```python
from build123d import *

# Parameters (mm, degrees)
ESQUISSE1_R             = 50
BOSS_EXTRU_1_DEPTH      = 10
ESQUISSE2_R             = 47.5
ENL_V_MAT_EXTRU_1_DEPTH = 5
ESQUISSE3_R             = 2
ENL_V_MAT_EXTRU_2_DEPTH = 5
BOSS_EXTRU_2_DEPTH      = 100
CONG_1_R                = 30
ESQUISSE5_R             = 12.5
BOSS_EXTRU_3_DEPTH      = 11
ENL_V_START             = -11
ESQUISSE6_R             = 2
ENL_V_MAT_EXTRU_3_DEPTH = 11


with BuildPart() as part:
    # Esquisse1 → Boss.-Extru.1 (new body)
    with BuildSketch(Plane.XY):
        Circle(ESQUISSE1_R)
    extrude(amount=BOSS_EXTRU_1_DEPTH)

    # Esquisse2 → Enlèv. mat.-Extru.1 (cut)
    with BuildSketch(Plane.XY.offset(10)):
        Circle(ESQUISSE2_R)
    extrude(amount=-ENL_V_MAT_EXTRU_1_DEPTH, mode=Mode.SUBTRACT)

    # Esquisse3 → Enlèv. mat.-Extru.2 (cut)
    with BuildSketch(Plane(origin=(0, 0, 0), x_dir=(-1, 0, 0), z_dir=(0, 0, -1))):
        Circle(ESQUISSE3_R)
    extrude(amount=-ENL_V_MAT_EXTRU_2_DEPTH, mode=Mode.SUBTRACT)

    # Esquisse4 → Boss.-Extru.2 (add)
    with BuildSketch(Plane(origin=(0, 0, 0), x_dir=(-1, 0, 0), z_dir=(0, 0, -1))):
        with BuildLine():
            ThreePointArc((-22.5, -30), (-37.5, 0), (-22.5, 30))
            Line((-22.5, 30), (-36.827299657, 30))
            ThreePointArc((-36.827299657, 30), (-47.5, 0), (-36.827299657, -30))
            Line((-36.827299657, -30), (-22.5, -30))
        make_face()
        with BuildLine():
            Line((36.827299657, 30), (22.5, 30))
            ThreePointArc((22.5, 30), (33.541019662, 16.770509831), (37.5, 0))
            ThreePointArc((37.5, 0), (33.541019662, -16.770509831), (22.5, -30))
            Line((22.5, -30), (36.827299657, -30))
            ThreePointArc((36.827299657, -30), (44.752355992, -15.920949505), (47.5, 0))
            ThreePointArc((47.5, 0), (44.752355992, 15.920949505), (36.827299657, 30))
        make_face()
    extrude(amount=BOSS_EXTRU_2_DEPTH)

    # Congé1
    # the kernel refuses this fillet: 30 mm, written as the material it takes off along each edge
    with BuildSketch(Plane(origin=(111.827299657, -30, -100), x_dir=(0, 0, 1), z_dir=(-1, 0, 0)), Plane(origin=(-52.5, 30, -100), x_dir=(0, 0, 1), z_dir=(1, 0, 0)), Plane(origin=(52.5, -30, -100), x_dir=(0, 0, 1), z_dir=(-1, 0, 0)), Plane(origin=(-111.827299657, 30, -100), x_dir=(0, 0, 1), z_dir=(1, 0, 0))) as cong_1_piece_1:
        with BuildLine():
            CenterArc((CONG_1_R, CONG_1_R), CONG_1_R, 180, 90)
            Line((0, CONG_1_R), (0, 0))
            Line((0, 0), (CONG_1_R, 0))
        make_face()
    extrude(amount=164.327299657, mode=Mode.SUBTRACT)

    # Esquisse5 → Boss.-Extru.3 (add)
    with BuildSketch(Plane.XY.offset(5)):
        Circle(ESQUISSE5_R)
    extrude(amount=BOSS_EXTRU_3_DEPTH)

    # Esquisse6 → Enlèv. mat.-Extru.3 (cut)
    with BuildSketch(Plane.XY.offset(16).offset(ENL_V_START)):
        with Locations(Location((0, 0, 0), (0, 0, 180))):
            Circle(ESQUISSE6_R)
    extrude(amount=ENL_V_MAT_EXTRU_3_DEPTH, mode=Mode.SUBTRACT)


solid = part.part
```
Geometry check sheet. Reference: the model listing, model coordinates, mm. A direction names the side the tool comes from. Round coordinates to 2 decimals unless told otherwise and drop trailing zeros. Order: outer loops, then holes, each group sorted by start corner. A loop starts at its lowest first (then second) coordinate and runs counter-clockwise, first axis right, second up. Notation, with made-up numbers: (18.5, 57) -> (51.5, 57) arc R11 ccw to (51.5, 69) -> close; hole circle Ø4 at (77.5, 32.5). An arc over 180 degrees is marked (long way). Return JSON: item names as keys, results as strings. Group by question number.
Q1. Gauge pin test, flat ends, axial feed: pin 1 (4 mm diameter, centred on x = 38.5, z = -28.5, fed in from -Y); pin 2 (1 mm diameter, centred on x = 26.5, y = -3.5, fed in from +Z); pin 3 (6.5 mm diameter, centred on x = 0, y = 0, fed in from -Z). Record the tip position at first contact, or that the pin passes through.
Q2. Section check C-C, the plane y = -21. Record the boundary of the cut face in (x, z), plus the area to 3 significant figures.
Q3. Material ranges on probe 1 along Y at (x, z) = (0, 7); probe 2 along Y at (x, z) = (0, 12); probe 3 along X at (y, z) = (29, -49), recorded low to high. Write a range as from..to.
Q4. Tool access check on faces 1 (the flat face through (-30, 30, -35)), 2 (the flat face through (30, -30, -35)), 3 (the cylindrical face through (47.498, 0.455, -49.303)), 4 (the flat face through (44.2, -18.3, 10)). Record the directions out of +Z, -Z, +X, -X, +Y, -Y that give a thin tool (end or side, any length) a straight path to the whole face; none if there is none.
Q5. Section check D-D, the plane x = 31. Record the boundary of the cut face in (y, z).
Q6. Section check A-A, the plane x = 0. Record the boundary of the cut face in (y, z), plus the area to 3 significant figures.
Q7. Section check B-B, the plane z = -57. Record the boundary of the cut face in (x, y), plus the area to 3 significant figures.
Numbers:
{
 "1": {"pin 1": "y = -30", "pin 2": "z = 5", "pin 3": "z = 0"},
 "2": {"outline": "(-45.38, 0) -> (-42.61, 0) -> (-42.61, -91.42) -> (-31.07, -91.42) -> (-31.07, 0) -> (31.07, 0) -> (31.07, -91.42) -> (42.61, -91.42) -> (42.61, 0) -> (45.38, 0) -> (45.38, 10) -> (42.61, 10) -> (42.61, 5) -> (-42.61, 5) -> (-42.61, 10) -> (-45.38, 10) -> close", "area": "2,590 mm^2"},
 "3": {"probe 1": "-50..-47.5, -12.5..-2, 2..12.5, 47.5..50", "probe 2": "-12.5..-2, 2..12.5", "probe 3": "-37.62..-23.77, 23.77..37.62"},
 "4": {"face 1": "-Z, +X, -X, +Y", "face 2": "-Z, +X, -X, -Y", "face 3": "-Z, +X", "face 4": "+Z"},
 "5": {"outline": "(-39.23, 0) -> (-30, 0) -> (-30, -70) arc R30 ccw to (-21.1, -91.32) -> (-21.1, 0) -> (21.1, 0) -> (21.1, -91.32) arc R30 ccw to (30, -70) -> (30, 0) -> (39.23, 0) -> (39.23, 10) -> (35.99, 10) -> (35.99, 5) -> (-35.99, 5) -> (-35.99, 10) -> (-39.23, 10) -> close"},
 "6": {"outline": "(-50, 0) -> (-2, 0) -> (-2, 16) -> (-12.5, 16) -> (-12.5, 5) -> (-47.5, 5) -> (-47.5, 10) -> (-50, 10) -> close; (2, 0) -> (50, 0) -> (50, 10) -> (47.5, 10) -> (47.5, 5) -> (12.5, 5) -> (12.5, 16) -> (2, 16) -> close", "area": "736 mm^2"},
 "7": {"outline": "(-36.83, -30) -> (-22.5, -30) arc R37.5 cw to (-22.5, 30) -> (-36.83, 30) arc R47.5 ccw to start; (22.5, -30) -> (36.83, -30) arc R47.5 ccw to (36.83, 30) -> (22.5, 30) arc R37.5 cw to start", "area": "1,340 mm^2"}
}
